Read the model definition and answer for the solid it produces. Units are mm, in the model's axes. A direction names the side the tool comes from. Round coordinates to 2 decimals unless told otherwise and drop trailing zeros. Loops run counter-clockwise (first coordinate to the right, second up) from the corner with the lowest first, then second, coordinate; pieces in that order, holes last. Notation, with made-up numbers: (55, 28) -> (60, 28) arc R32 cw to (60, 65) -> close; hole circle Ø3 at (-25, 21). An arc over 180 degrees is marked (long way). Put each result on its own line as item: value.
from build123d import *

# Parameters (mm, degrees)
SKETCH005_W              = 0.5
SKETCH005_H              = 0.5
SKETCH006_W              = 0.5
SKETCH006_H              = 0.5
ADDITIVEPIPE001_FACE21_W = 0.5
ADDITIVEPIPE001_FACE21_H = 0.5
PAD001_DEPTH             = 3
POCKET_DEPTH             = 5


with BuildPart() as part:
    # Sketch002 → Revolution (revolve)
    with BuildSketch(Plane.XY):
        with BuildLine():
            Line((0, 2.45), (-5.55, 2.45))
            Line((-5.55, 2.45), (-5.55, 3))
            Line((-5.55, 3), (-6.55, 3))
            Line((-6.55, 3), (-6.55, 0))
            Line((2.45, 0), (-6.55, 0))
            ThreePointArc((2.45, 0), (1.732412, 1.732412), (0, 2.45))
        make_face()
    revolve(axis=Axis((0, 0, 0), (1, 0, 0)))

    # AdditivePipe: sweep along a path in Sketch004
    with BuildLine(Plane.XZ) as additivepipe_path:
        Line((-6.55, 0), (-6.65, 0))
        ThreePointArc((-6.65, 0), (-7.357107, -0.292893), (-7.65, -1))
        Line((-7.65, -1), (-7.65, -15))
    # Sketch005 (on Face4 of Revolution) → AdditivePipe (sweep)
    with BuildSketch(Plane(origin=(-6.55, 0, 0), x_dir=(0, -1, 0), z_dir=(-1, 0, 0))):
        with Locations((1.25, 0)):
            Rectangle(SKETCH005_W, SKETCH005_H)
    sweep(path=additivepipe_path.line)

    # AdditivePipe001: sweep along a path in Sketch004
    with BuildLine(Plane.XZ) as additivepipe001_path:
        Line((-6.55, 0), (-6.65, 0))
        ThreePointArc((-6.65, 0), (-7.357107, -0.292893), (-7.65, -1))
        Line((-7.65, -1), (-7.65, -15))
    # Sketch006 (on Face4 of Revolution) → AdditivePipe001 (sweep)
    with BuildSketch(Plane(origin=(-6.55, 0, 0), x_dir=(0, -1, 0), z_dir=(-1, 0, 0))):
        with Locations((-1.25, 0)):
            Rectangle(SKETCH006_W, SKETCH006_H)
    sweep(path=additivepipe001_path.line)

    # AdditivePipe001 Face21 → Pad001 (new)
    with BuildSketch(Plane(origin=(-7.65, 1.25, -15), x_dir=(0, -1, 0), z_dir=(0, 0, -1))):
        Rectangle(ADDITIVEPIPE001_FACE21_W, ADDITIVEPIPE001_FACE21_H)
    extrude(amount=PAD001_DEPTH)

    # Sketch007 (on Face3 of Pad001) → Pocket (cut)
    with BuildSketch(Plane.YZ.offset(-5.55)):
        with BuildLine():
            Line((-2.45, 1.731329), (-2.45, -1.731329))
            ThreePointArc((-2.45, 1.731329), (-3.000002, 0), (-2.45, -1.731329))
        make_face()
    extrude(amount=-POCKET_DEPTH, mode=Mode.SUBTRACT)


solid = part.part
Item 1: The part is cut by section D-D (z = -1.5). State how many separate pieces and enclosed holes the cut face has, then the cut area to 3 significant figures.
Derived:
separate pieces: 3
enclosed holes: 0
area: 32.9 mm^2
Item 2: The part is cut by section B-B (x = -2.25). Determine the outline of the cut face in (y, z).
Derived:
outline: circle Ø4.9 at (0, 0)
Item 3: Which of the six approach directions +Z, -Z, +X, -X, +Y, -Y give full straight-line access (tool end or side, diameter ignored) to faces 4 (the flat face through (-6, -2.45, 0)), 5 (the flat face through (-7.6, 1, -8.8)), 6 (the flat face through (-5.55, 2, 2)), 7 (the flat face through (-7.6, -1.5, -7.4)), 8 (the cylindrical face through (-7.524, 1.253, -0.106))?
Derived:
face 4: +Z, -Z, +X, -X, -Y
face 5: +Z, -Z, -X
face 6: +X
face 7: +Z, -Z, -X, -Y
face 8: +Z, -X, +Y, -Y
Item 4: Flat-ended cylindrical pins translate along their axes: pin 1 Ø1.5 at (x, y) = (-0.5, 1.5) entering from +Z; pin 2 Ø1.5 at (x, z) = (-7, -9) entering from +Y; pin 3 Ø2 at (x, y) = (-3.5, -0.5) entering from -Z. Find the tip coordinate at first contact, or state that the pin passes through.
Derived:
pin 1: stops at z = 2.33
pin 2: stops at y = 1.5
pin 3: stops at z = -2.45
Item 5: The part is cut by section A-A (z = -10). Determine the outline of the cut face in (x, y).
Derived:
outline: (-7.9, -1.5) -> (-7.4, -1.5) -> (-7.4, -1) -> (-7.9, -1) -> close; (-7.9, 1) -> (-7.4, 1) -> (-7.4, 1.5) -> (-7.9, 1.5) -> close
Item 6: The part is cut by section C-C (z = -16). Determine the outline of the cut face in (x, y), then the cut area to 3 significant figures.
Derived:
outline: (-7.9, 1) -> (-7.4, 1) -> (-7.4, 1.5) -> (-7.9, 1.5) -> close
area: 0.250 mm^2
Item 7: Find the intervals of material crossed by line 1 along X through (y, z) = (-1.4, -2.25); line 2 along X through (y, z) = (-0.9, -2.75); line 3 along X through (y, z) = (1.05, -12.5), in increasing order.
Derived:
line 1: x = -7.9 to -7.4, -6.55 to -5.55
line 2: x = -6.55 to -5.55
line 3: x = -7.9 to -7.4
Item 8: For a pull along Y with two mould halves and no side action, classify faces 1 (the flat face through (-7.6, 1.5, -8.8)), 2 (the flat face through (-7.7, -1, -7.3)), 3 (the cylindrical face through (-7.524, -1.246, -0.106)) as pulls with the +Y half, pulls with the -Y half, needs draft (parallel to the pull), parting line crosses it, or undercut.
Derived:
face 1: pulls with the +Y half
face 2: undercut
face 3: needs draft
